Part model, mm, in its own coordinate system. Face numbers are marked on the shaded views. A direction names the side the tool comes from. Round coordinates to 2 decimals unless told otherwise and drop trailing zeros. Order: outer loops, then holes, each group sorted by start corner. A loop starts at its lowest first (then second) coordinate and runs counter-clockwise, first axis right, second up. Notation, with made-up numbers: (-11.5, -6.5) - (41.5, -6.5) arc R12 cw to (41.5, -0.5) - close; hole circle Ø4 at (51.25, 53.5). An arc over 180 degrees is marked (long way). Return JSON: item names as keys, results as strings. Group by question number.
Item 1: Saw through at D-D on z = 14. List the corners of the cut face in (x, y).
Item 2: Probe probe 1 along Y at (x, z) = (0, 10.2); probe 2 along Y at (x, z) = (0, 5.75); probe 3 along X at (y, z) = (-2, 8.5). List the from-to ranges inside material, lowest first.
Item 3: Drop flat-ended pins along their axis: pin 1 (16.5 mm diameter, centred on x = 0, y = 0, fed in from -Z); pin 2 (6 mm diameter, centred on x = -6, z = 12.5, fed in from +Y); pin 3 (3 mm diameter, centred on y = -12, z = 11, fed in from +X); pin 4 (6 mm diameter, centred on y = 11, z = 2.5, fed in from +X). Give the stop position or say it passes through.
Item 4: Tool access for the marked faces 1 and 2: list every direction of +Z, -Z, +X, -X, +Y, -Y with a clear straight run to the whole face (end or side of a thin tool).
Item 5: Saw through at A-A on x = 0. List the corners of the cut face in (y, z), and give its area (3 significant figures).
Item 6: Two-plate mould, pull along X, no slides. Class the marked faces 3, 4 and 5: released by +X, released by -X, zero draft, split by the parting line, or undercut.
Item 7: Saw through at B-B on z = 12. List the corners of the cut face in (x, y), and give its area (3 significant figures).
```python
from build123d import *

# Parameters (mm, degrees)
F0_R     = 16.51
F0_R_2   = 10.1780603176
F1_DEPTH = 15.24
F0_R_3   = 3.9258092534
F0_R_4   = 1.27
F2_DEPTH = 7.62
F3_R     = 2.54


with BuildPart() as f1:
    # F0 (on Top) → F1 (new body)
    with BuildSketch(Plane.XY):
        Circle(F0_R)
        Circle(F0_R_2, mode=Mode.SUBTRACT)
    extrude(amount=F1_DEPTH)



with BuildPart() as f1b:
    # F0 (on Top) → F1, piece 2 (new body)
    with BuildSketch(Plane.XY):
        Circle(F0_R_3)
        Circle(F0_R_4, mode=Mode.SUBTRACT)
    extrude(amount=F1_DEPTH)


with BuildPart() as f1_1:
    add(f1.part)

    add(f1b.part)  # F2 merges F1b
    # F0 (on Top) → F2 (join)
    with BuildSketch(Plane.XY):
        Circle(F0_R_2)
        Circle(F0_R_3, mode=Mode.SUBTRACT)
    extrude(amount=F2_DEPTH)

    # F3
    f3_edges = [f1_1.edges().sort_by_distance(p)[0] for p in [
        (-16.51, 0, 15.24),
        (-16.51, 0, 0),
        (-10.17806, 0, 15.24),
    ]]
    fillet(f3_edges, radius=F3_R)


solid = f1_1.part
```
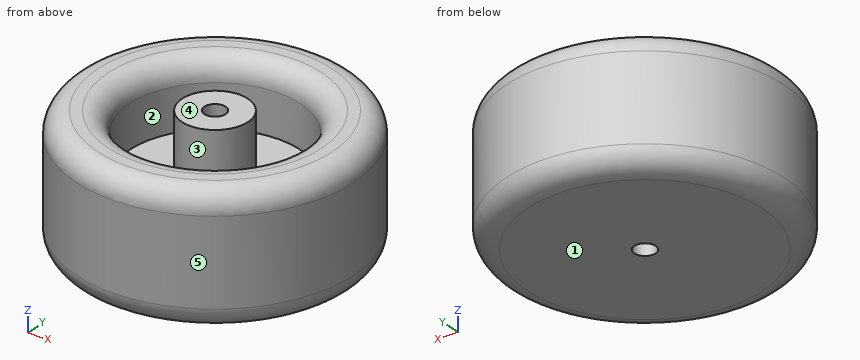
Filled in:
{
 "1": {"outline": "circle Ø32.3 at (0, 0); circle Ø7.85 at (0, 0); hole circle Ø21.07 at (0, 0); hole circle Ø2.54 at (0, 0)"},
 "2": {"probe 1": "y = -16.51 to -10.18, -3.93 to -1.27, 1.27 to 3.93, 10.18 to 16.51", "probe 2": "y = -16.51 to -1.27, 1.27 to 16.51", "probe 3": "x = -16.39 to -9.98, -3.38 to 3.38, 9.98 to 16.39"},
 "3": {"pin 1": "stops at z = 0", "pin 2": "stops at y = 16.24", "pin 3": "stops at x = 12.74", "pin 4": "stops at x = 14.44"},
 "4": {"face 1": "-Z, +X, -X, +Y, -Y", "face 2": "+Z"},
 "5": {"outline": "(-16.51, 2.54) arc R2.54 ccw to (-13.97, 0) - (-1.27, 0) - (-1.27, 15.24) - (-3.93, 15.24) - (-3.93, 7.62) - (-10.18, 7.62) - (-10.18, 12.7) arc R2.54 ccw to (-12.72, 15.24) - (-13.97, 15.24) arc R2.54 ccw to (-16.51, 12.7) - close; (1.27, 0) - (13.97, 0) arc R2.54 ccw to (16.51, 2.54) - (16.51, 12.7) arc R2.54 ccw to (13.97, 15.24) - (12.72, 15.24) arc R2.54 ccw to (10.18, 12.7) - (10.18, 7.62) - (3.93, 7.62) - (3.93, 15.24) - (1.27, 15.24) - close", "area": "361 mm^2"},
 "6": {"face 3": "undercut", "face 4": "zero draft", "face 5": "split by the parting line"},
 "7": {"outline": "circle Ø33.02 at (0, 0); circle Ø7.85 at (0, 0); hole circle Ø20.36 at (0, 0); hole circle Ø2.54 at (0, 0)", "area": "574 mm^2"}
}
